Could you check a few things on this model? Use its own coordinates, in mm. A direction names the side the tool comes from. Give positions to 0.01 mm unless a question says otherwise; leave off trailing zeros. Loops run counter-clockwise (first coordinate to the right, second up) from the corner with the lowest first, then second, coordinate; pieces in that order, holes last. Notation, with made-up numbers: (-20.5, 30.25) - (-8.5, 30.25) arc R28 ccw to (-8.5, 57.25) - close; hole circle Ø1 at (50.25, 26). An arc over 180 degrees is marked (long way). Write each question's results on one line, items separated by ' | '. Start each with the question number.
(1) Suppose I cut it at D-D (z = 13). Please give me the cut outline in (x, y), and give its area (3 significant figures).
(2) I need wall thicknesses on line 1 (Z direction, x = 67.5, y = 31); line 2 (X direction, y = 25, z = 5); line 3 (Y direction, x = 32, z = 24.5). Which ranges of each line are inside material? Lowest first, please.
(3) Suppose I cut it at B-B (y = 14). Please give me the cut outline in (x, z), and give its area (3 significant figures).
(4) On a 3-axis mill with a long thin cutter (end or side, diameter ignored), from which of +Z, -Z, +X, -X, +Y, -Y can I reach the whole of each face in a straight line? I mean faces 4 (the face through (3, 32, 12)), 5 (the face through (79, 25, 40)), 6 (the face through (41.038, -11.404, 28.224)). Say none if no direction works.
(5) Suppose I cut it at A-A (z = 38.5). Please give me the cut outline in (x, y).
(6) Suppose I cut it at C-C (x = 4). Please give me the cut outline in (y, z), and give its area (3 significant figures).
(7) For pin 1 (12 mm diameter, centred on y = 6, z = 33.5, fed in from -X); pin 2 (8 mm diameter, centred on y = -4.5, z = 28.5, fed in from -X); pin 3 (1.5 mm diameter, centred on y = 29, z = 25.5, fed in from -X), each with a flat end and sliding along its axis, tell me the tip position at first contact or that it passes through.
(8) If we mould it in two halves opening along Y, with no side actions, what happens to faces 1 (the face through (75.824, 35.762, 40.549)), 2 (the face through (76, 37, 6)), 3 (the face through (-7, 16, 12))? For each: released by +Y, released by -Y, zero draft, split by the parting line, or undercut.
from build123d import *

# Parameters (mm, degrees)
SKETCH1_R           = 7
BOSS_EXTRUDE1_DEPTH = 44
SKETCH70_W          = 24
SKETCH70_H          = 39.86554544
SKETCH71_W          = 34
SKETCH71_H          = 19
CUT_EXTRUDE1_DEPTH  = 43
SKETCH73_R          = 5.5
CUT_EXTRUDE3_DEPTH  = 99.478424033
CUT_EXTRUDE4_DEPTH  = 32
SKETCH78_14_R       = 5.5
CUT_EXTRUDE5_DEPTH  = 7


with BuildPart() as part:
    # Sketch1 → Boss-Extrude1 (new body)
    with BuildSketch(Plane.XY):
        with BuildLine():
            Line((0, 0), (-7, 7))
            Line((-7, 7), (-7, 25))
            Line((-7, 25), (0, 32))
            Line((0, 32), (6.423127039, 32))
            Line((6.423127039, 32), (29.319429923, 27.962764043))
            ThreePointArc((29.319429923, 27.962764043), (41.564716358, 29.911963462), (50, 39))
            Line((50, 39), (74, 39))
            Line((74, 39), (79, 34))
            Line((79, 34), (79, 15))
            Line((79, 15), (50, -19))
            Line((50, -19), (44.788067397, -19))
            ThreePointArc((44.788067397, -19), (40.27095427, -12.128573817), (37.89327269, -4.256633834))
            ThreePointArc((37.89327269, -4.256633834), (36.210984968, -1.21075002), (32.948840798, 0))
            Line((32.948840798, 0), (0, 0))
        make_face()
        with Locations((7, 14)):
            Circle(SKETCH1_R, mode=Mode.SUBTRACT)
    extrude(amount=BOSS_EXTRUDE1_DEPTH)

    # Sketch70 → Cut-Revolve3 (revolve, cut)
    with BuildSketch(Plane(origin=(79, 0, 0), x_dir=(0, 0, -1), z_dir=(1, 0, 0))):
        with Locations((-24, 19.06722728)):
            Rectangle(SKETCH70_W, SKETCH70_H)
    revolve(axis=Axis((79, 39, 36), (0, 0, -1)), mode=Mode.SUBTRACT)

    # Sketch71 → Cut-Extrude1 (cut)
    with BuildSketch(Plane(origin=(0, 39, 0), x_dir=(1, 0, 0), z_dir=(0, 1, 0))):
        with Locations((10, -34.5)):
            Rectangle(SKETCH71_W, SKETCH71_H)
    extrude(amount=-CUT_EXTRUDE1_DEPTH, mode=Mode.SUBTRACT)

    # Sketch73 → Cut-Extrude3 (cut, through all)
    with BuildSketch(Plane.XY):
        with Locations(Location((65, 25, 0), (0, 0, 180))):
            Circle(SKETCH73_R)
    extrude(amount=CUT_EXTRUDE3_DEPTH, mode=Mode.SUBTRACT)

    # Sketch78 → Cut-Extrude4 (cut)
    with BuildSketch(Plane.XY.offset(44)):
        with BuildLine():
            ThreePointArc((36.944123049, 27.147434538), (33.053294732, 26.678832738), (29.145781746, 26.97795629))
            Line((29.145781746, 26.97795629), (28, 27.179988526))
            Line((28, 27.179988526), (28, 1))
            Line((28, 1), (32.948840798, 1))
            ThreePointArc((32.948840798, 1), (36.863413802, -0.452900023), (38.882159069, -4.107960601))
            ThreePointArc((38.882159069, -4.107960601), (41.083042895, -11.502353322), (45.242552598, -18))
            Line((45.242552598, -18), (49.538593943, -18))
            Line((49.538593943, -18), (65.164712554, 0.320276992))
            ThreePointArc((65.164712554, 0.320276992), (47.987855004, 10.508012336), (36.944123049, 27.147434538))
        make_face()
    extrude(amount=-CUT_EXTRUDE4_DEPTH, mode=Mode.SUBTRACT)

    # Sketch78_14 → Cut-Extrude5 (cut)
    with BuildSketch(Plane.XY.offset(44)):
        with BuildLine():
            ThreePointArc((50.639838281, 38), (45.039926113, 30.998835685), (36.944123049, 27.147434538))
            ThreePointArc((36.944123049, 27.147434538), (47.987855004, 10.508012336), (65.164712554, 0.320276992))
            Line((65.164712554, 0.320276992), (78, 15.368545033))
            Line((78, 15.368545033), (78, 33.585786438))
            Line((78, 33.585786438), (73.585786438, 38))
            Line((73.585786438, 38), (50.639838281, 38))
        make_face()
        with Locations((65, 25)):
            Circle(SKETCH78_14_R, mode=Mode.SUBTRACT)
    extrude(amount=-CUT_EXTRUDE5_DEPTH, mode=Mode.SUBTRACT)


solid = part.part
Output values:
1) outline: (-7, 7) - (0, 0) - (32.95, 0) arc R5 cw to (37.89, -4.26) arc R28.63 ccw to (44.79, -19) - (50, -19) - (67.04, 0.97) arc R39.87 cw to (40.33, 29.31) arc R19 cw to (29.32, 27.96) - (6.42, 32) - (0, 32) - (-7, 25) - close; hole circle Ø14 at (7, 14); hole (28, 1) - (32.95, 1) arc R6 cw to (38.88, -4.11) arc R27.63 ccw to (45.24, -18) - (49.54, -18) - (65.16, 0.32) arc R44.8 cw to (36.94, 27.15) arc R20 cw to (29.15, 26.98) - (28, 27.18) - close | area: 1,040 mm2
2) line 1: 0 to 12, 36 to 37 | line 2: -7 to 59.5, 70.5 to 79 | line 3: 0 to 1, 26.68 to 27.68
3) outline: (-7, 0) - (0, 0) - (0, 25) - (-7, 25) - close; (14, 0) - (78.15, 0) - (78.15, 12) - (47.95, 12) - (47.95, 36) - (78.15, 36) - (78.15, 44) - (76.83, 44) - (76.83, 37) - (44.69, 37) - (44.69, 12) - (28, 12) - (28, 44) - (27, 44) - (27, 25) - (14, 25) - close | area: 1,270 mm2
4) face 4: +Z, -Z, -X, +Y | face 5: +Z, -Z, +X, +Y, -Y | face 6: +Z
5) outline: (27, 0) - (32.95, 0) arc R5 cw to (37.89, -4.26) arc R28.63 ccw to (44.79, -19) - (50, -19) - (79, 15) - (79, 34) - (74, 39) - (50, 39) arc R19 cw to (29.32, 27.96) - (27, 28.37) - close; hole (28, 1) - (32.95, 1) arc R6 cw to (38.88, -4.11) arc R27.63 ccw to (45.24, -18) - (49.54, -18) - (78, 15.37) - (78, 33.59) - (73.59, 38) - (50.64, 38) arc R20 cw to (29.15, 26.98) - (28, 27.18) - close
6) outline: (0, 0) - (7.68, 0) - (7.68, 25) - (0, 25) - close; (20.32, 0) - (32, 0) - (32, 25) - (20.32, 25) - close | area: 484 mm2
7) pin 1: x = 27 | pin 2: x = 35.13 | pin 3: x = -3.56
8) face 1: undercut | face 2: released by +Y | face 3: zero draft
